Geometry: see drawing. Coordinates: mm, zero at the bounding-box minimum. A direction names the side the tool comes from. Give positions to 0.01 mm unless a question says otherwise; leave off trailing zeros. Order: outer loops, then holes, each group sorted by start corner. A loop starts at its lowest first (then second) coordinate and runs counter-clockwise, first axis right, second up. Notation, with made-up numbers: M 7,55 L 40,55 A29 cw 40,81 Z; hole C 17,67 d4. An arc over 180 degrees is marked long. Answer as a JSON object with one key per item and string values. Group by question number.
1. Pin query (flat end, axial travel): P1, Ø1, axis at x = 59.5, y = 5.5, coming from the +Z side; P2, Ø4, axis at x = 49, y = 8.5, coming from the -Z side (1 decimal); P3, Ø2, axis at x = 33.5, z = 27, coming from the -Y side (3 decimals). Return the tip coordinate at first contact, or that it passes through.
2. Section query D-D (y = 2). Output: boundary loops of the cut face in (x, z) (3 decimals), plus the area to 3 significant figures.
3. Section query C-C (x = 27). Output: boundary loops of the cut face in (y, z) (1 decimal), plus the area to 3 significant figures.
4. Section query A-A (z = 82.55). Output: boundary loops of the cut face in (x, y) (3 decimals).
5. Section query B-B (z = 120.65). Count the separate pieces of the cut face and the enclosed holes in it, plus the area to 3 significant figures.
6. Set-up query: the marked faces 1 and 2. Return all of +Z, -Z, +X, -X, +Y, -Y with unobstructed straight access to the full face (end or side cutting, diameter ignored); none if empty.
7. Material intervals for L1, parallel to Z at x = 82.55, y = 12; L2, parallel to Z at x = 82.55, y = 5.5 (3 decimals); L3, parallel to X at y = 12, z = 83.5, sorted ascending. Write a range as [from, to].
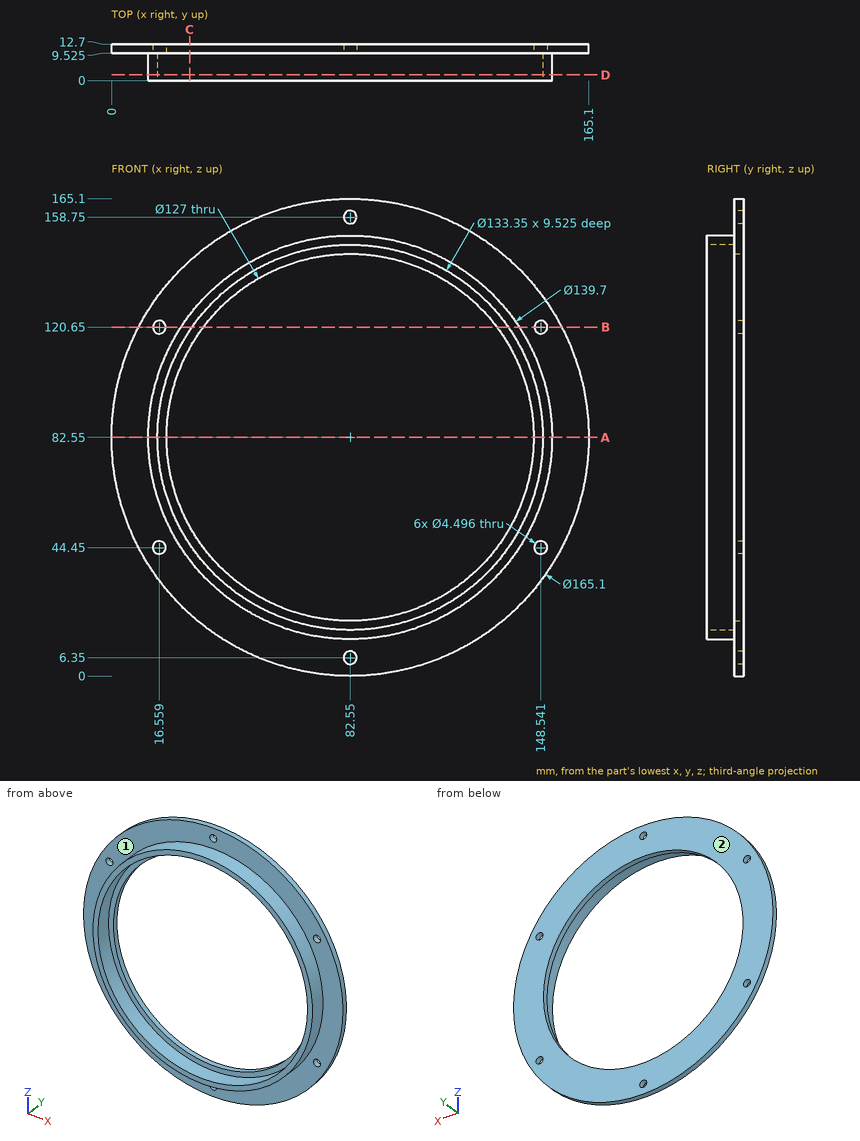
Answer sheet:
{
 "1": {"P1": "z = 148.66", "P2": "z = 6.4", "P3": "y = 9.525"},
 "2": {"outline": "C 82.55,82.55 d139.7; hole C 82.55,82.55 d133.35", "area": "1,360 mm^2"},
 "3": {"outline": "M 0,40.2 L 9.5,40.2 L 9.5,21.5 L 12.7,21.5 L 12.7,51.8 L 9.5,51.8 L 9.5,45.7 L 0,45.7 Z; M 0,119.4 L 9.5,119.4 L 9.5,113.3 L 12.7,113.3 L 12.7,143.6 L 9.5,143.6 L 9.5,124.9 L 0,124.9 Z", "area": "297 mm^2"},
 "4": {"outline": "M 0,9.525 L 12.7,9.525 L 12.7,0 L 15.875,0 L 15.875,9.525 L 19.05,9.525 L 19.05,12.7 L 0,12.7 Z; M 146.05,9.525 L 149.225,9.525 L 149.225,0 L 152.4,0 L 152.4,9.525 L 165.1,9.525 L 165.1,12.7 L 146.05,12.7 Z"},
 "5": {"separate pieces": "4", "enclosed holes": "0", "area": "187 mm^2"},
 "6": {"face 1": "-Y", "face 2": "+Z, -Z, +X, -X, +Y"},
 "7": {"L1": "[0, 4.1], [8.6, 19.05], [146.05, 156.5], [161, 165.1]", "L2": "[12.7, 15.875], [149.225, 152.4]", "L3": "[0.01, 19.06], [146.04, 165.09]"}
}
